Can you work these out from the model? Positions are in its coordinate system, mm. A direction names the side the tool comes from. Coordinates: 2 decimals unless noted, no trailing zeros. Loops run counter-clockwise (first coordinate to the right, second up) from the corner with the lowest first, then second, coordinate; pieces in that order, holes last.
```python
from build123d import *

# Parameters (mm, degrees)
CUT_EXTRUDE1_DEPTH = 4.7


with BuildPart() as part:
    # Sketch1 → Revolve1 (revolve)
    with BuildSketch(Plane(origin=(0, 0, 0), x_dir=(0, 0, -1), z_dir=(1, 0, 0))):
        with BuildLine():
            Line((-21.5, 0), (-21.5, 5.8))
            Line((-21.5, 5.8), (-21.3, 6))
            Line((-21.3, 6), (-16.2, 6))
            ThreePointArc((-16.2, 6), (-15.917157288, 6.117157288), (-15.8, 6.4))
            Line((-15.8, 6.4), (-15.8, 12.66))
            Line((-15.8, 12.66), (-15.5, 12.96))
            Line((-15.5, 12.96), (-6.1, 12.96))
            ThreePointArc((-6.1, 12.96), (-5.887867966, 13.047867966), (-5.8, 13.26))
            Line((-5.8, 13.26), (405, 13.26))
            Line((405, 13.26), (405, 20))
            Line((405, 20), (415, 20))
            Line((415, 20), (415, 0))
            Line((415, 0), (-21.5, 0))
        make_face()
    revolve(axis=Axis((0, 0, -415), (0, 0, 1)))

    # Sketch2 → Revolve2 (revolve)
    with BuildSketch(Plane(origin=(0, 0, 0), x_dir=(0, 0, -1), z_dir=(1, 0, 0))):
        with BuildLine():
            Line((-40.5, 0), (-40.5, 4.233))
            Line((-40.5, 4.233), (-39.733, 5))
            Line((-39.733, 5), (-24.332050808, 5))
            Line((-24.332050808, 5), (-22.739230485, 4.080384758))
            ThreePointArc((-22.739230485, 4.080384758), (-22.594521912, 4.020444504), (-22.439230485, 4))
            Line((-22.439230485, 4), (-22.1, 4))
            ThreePointArc((-22.1, 4), (-21.675735931, 4.175735931), (-21.5, 4.6))
            Line((-21.5, 4.6), (-21.5, 0))
            Line((-21.5, 0), (-40.5, 0))
        make_face()
    revolve(axis=Axis((0, 0, 21.5), (0, 0, 1)))

    # Sketch3 → Cut-Extrude1 (cut)
    with BuildSketch(Plane.XY.offset(21.5)):
        Polygon((-7, 8), (-7, -6), (-5, -6), (-5, 6), (5, 6), (5, -6), (7, -6), (7, 8), align=None)
    extrude(amount=-CUT_EXTRUDE1_DEPTH, mode=Mode.SUBTRACT)


solid = part.part
```
Item 1: Suppose I cut it at A-A, the plane z = -288. Please give me the cut outline in (x, y).
Results are:
outline: circle Ø26.52 at (0, 0)
Item 2: I need wall thicknesses on line 1 along Z through (x, y) = (12, 5); line 2 along Z through (x, y) = (6, 14.5); line 3 along Y through (x, z) = (-4, -102). Which ranges of each line are inside material? Lowest first, please.
Results are:
line 1: z = -415 to 5.95
line 2: z = -415 to -405
line 3: y = -12.64 to 12.64
Item 3: I'm going to push flat-ended pins straight in: P1, Ø12, axis at y = 4, z = -302.5, coming from the -X side; P2, Ø4, axis at y = -1.5, z = 20, coming from the +X side; P3, Ø10, axis at x = 3, z = -256.5, coming from the -Y side. Where does each tip first touch, or does it pass through?
Results are:
P1: stops at x = -13.26
P2: stops at x = 5
P3: stops at y = -13.26
Item 4: We'd pull the mould along Z, two halves only. Please class faces 4 (the face through (4.88, -1.08, 31.92)), 5 (the face through (3, -4, 21.5)), 6 (the face through (0, 0, -415)): +Z half, -Z half, draft (parallel to the pull), parting line (faces both ways), or undercut.
Results are:
face 4: draft
face 5: undercut
face 6: -Z half
Item 5: On a 3-axis mill with a long thin cutter (end or side, diameter ignored), from which of +Z, -Z, +X, -X, +Y, -Y can I reach the whole of each face in a straight line? I mean faces 1 (the face through (0, -6, 19)), 2 (the face through (0, 0, 40.5)), 3 (the face through (3.905, -0.867, 22.267)). Say none if no direction works.
Results are:
face 1: +Z
face 2: +Z, +X, -X, +Y, -Y
face 3: none
